```python
from build123d import *

# Parameters (mm, degrees)
SKETCH1_W               = 212.5
SKETCH1_H               = 339.725
BOSS_EXTRUDE1_DEPTH     = 6
SKETCH2_W               = 6.5
SKETCH2_H               = 20
BOSS_EXTRUDE2_DEPTH     = 24
CUT_EXTRUDE1_DEPTH      = 393.36344838
CUT_EXTRUDE1_DEPTH_BACK = 393.36344838
SKETCH3_R               = 4
FILLET2_R               = 5
SKETCH5_R               = 3.175
CUT_EXTRUDE2_DEPTH      = 402.314497153
CUT_EXTRUDE3_DEPTH      = 402.314497153


with BuildPart() as part:
    # Sketch1 → Boss-Extrude1 (new body)
    with BuildSketch(Plane.XY):
        with Locations((106.25, -169.8625)):
            Rectangle(SKETCH1_W, SKETCH1_H)
    extrude(amount=BOSS_EXTRUDE1_DEPTH)

    # Sketch2 → Boss-Extrude2 (add)
    with BuildSketch(Plane.XY.offset(6)):
        with Locations((21.75, -35.2425)):
            Rectangle(SKETCH2_W, SKETCH2_H)
        with Locations((50.75, -35.2425)):
            Rectangle(SKETCH2_W, SKETCH2_H)
        with Locations((190.75, -35.2425)):
            Rectangle(SKETCH2_W, SKETCH2_H)
        with Locations((161.75, -35.2425)):
            Rectangle(SKETCH2_W, SKETCH2_H)
        with Locations((133.75, -104.5325)):
            Rectangle(SKETCH2_W, SKETCH2_H)
        with Locations((165.25, -104.5325)):
            Rectangle(SKETCH2_W, SKETCH2_H)
        with Locations((165.25, -235.1925)):
            Rectangle(SKETCH2_W, SKETCH2_H)
        with Locations((21.75, -304.4825)):
            Rectangle(SKETCH2_W, SKETCH2_H)
        with Locations((50.75, -304.4825)):
            Rectangle(SKETCH2_W, SKETCH2_H)
        with Locations((190.75, -304.4825)):
            Rectangle(SKETCH2_W, SKETCH2_H)
        with Locations((161.75, -304.4825)):
            Rectangle(SKETCH2_W, SKETCH2_H)
        with Locations((133.75, -235.1925)):
            Rectangle(SKETCH2_W, SKETCH2_H)
    extrude(amount=BOSS_EXTRUDE2_DEPTH)

    # Sketch3 → Cut-Extrude1 (cut, two sides: drawn at the far end of the back side and taken through both)
    with BuildSketch(Plane.ZY.offset(-18.5).offset(-CUT_EXTRUDE1_DEPTH_BACK)):
        with Locations(Location((18, -35.2425, 0), (0, 0, 180))):
            Circle(SKETCH3_R)
        with Locations((18, -235.1925)):
            Circle(SKETCH3_R)
        with Locations(Location((18, -304.4825, 0), (0, 0, 270))):
            Circle(SKETCH3_R)
        with Locations(Location((18, -104.5325, 0), (0, 0, 180))):
            Circle(SKETCH3_R)
        with BuildLine():
            Line((18, -25.2425), (18, -12.982943413))
            Line((18, -12.982943413), (51.949532367, -12.982943413))
            Line((51.949532367, -12.982943413), (51.949532367, -57.481006387))
            Line((51.949532367, -57.481006387), (18, -57.481006387))
            Line((18, -57.481006387), (18, -45.2425))
            ThreePointArc((18, -45.2425), (28, -35.2425), (18, -25.2425))
        make_face()
        with BuildLine():
            Line((52.442304634, -132.399123951), (18, -132.399123951))
            Line((18, -132.399123951), (18, -114.5325))
            ThreePointArc((18, -114.5325), (28, -104.5325), (18, -94.5325))
            Line((18, -94.5325), (18, -71.59149594))
            Line((18, -71.59149594), (52.442304634, -71.59149594))
            Line((52.442304634, -71.59149594), (52.442304634, -132.399123951))
        make_face()
        with BuildLine():
            Line((52.599532243, -270.375386727), (18, -270.375386727))
            Line((18, -270.375386727), (18, -245.1925))
            ThreePointArc((18, -245.1925), (28, -235.1925), (18, -225.1925))
            Line((18, -225.1925), (18, -207.306351849))
            Line((18, -207.306351849), (52.599532243, -207.306351849))
            Line((52.599532243, -207.306351849), (52.599532243, -270.375386727))
        make_face()
        with BuildLine():
            Line((52.621034016, -326.721115515), (18, -326.721115515))
            Line((18, -326.721115515), (18, -314.4825))
            ThreePointArc((18, -314.4825), (28, -304.4825), (18, -294.4825))
            Line((18, -294.4825), (18, -282.222834285))
            Line((18, -282.222834285), (52.621034016, -282.222834285))
            Line((52.621034016, -282.222834285), (52.621034016, -326.721115515))
        make_face()
    extrude(amount=CUT_EXTRUDE1_DEPTH + CUT_EXTRUDE1_DEPTH_BACK, mode=Mode.SUBTRACT)

    # Fillet2
    fillet2_edges = [part.edges().sort_by_distance(p)[0] for p in [
        (190.75, -45.2425, 6),
        (194, -35.2425, 6),
        (190.75, -25.2425, 6),
        (50.75, -45.2425, 6),
        (54, -35.2425, 6),
        (50.75, -25.2425, 6),
        (21.75, -25.2425, 6),
        (18.5, -35.2425, 6),
        (21.75, -45.2425, 6),
        (161.75, -25.2425, 6),
        (158.5, -35.2425, 6),
        (161.75, -45.2425, 6),
        (161.75, -294.4825, 6),
        (161.75, -314.4825, 6),
        (158.5, -304.4825, 6),
        (190.75, -314.4825, 6),
        (194, -304.4825, 6),
        (190.75, -294.4825, 6),
        (165.25, -245.1925, 6),
        (168.5, -235.1925, 6),
        (165.25, -225.1925, 6),
        (133.75, -225.1925, 6),
        (130.5, -235.1925, 6),
        (133.75, -245.1925, 6),
        (50.75, -314.4825, 6),
        (54, -304.4825, 6),
        (50.75, -294.4825, 6),
        (21.75, -294.4825, 6),
        (21.75, -314.4825, 6),
        (18.5, -304.4825, 6),
        (165.25, -114.5325, 6),
        (165.25, -94.5325, 6),
        (168.5, -104.5325, 6),
        (133.75, -94.5325, 6),
        (130.5, -104.5325, 6),
        (133.75, -114.5325, 6),
    ]]
    fillet(fillet2_edges, radius=FILLET2_R)

    # Sketch5 → Cut-Extrude2 (cut, through all)
    with BuildSketch(Plane.XY.offset(6)):
        with Locations((12.7, -12.7)):
            Circle(SKETCH5_R)
        with Locations((199.8, -12.7)):
            Circle(SKETCH5_R)
        with Locations((66.25, -35.2425)):
            Circle(SKETCH5_R)
        with Locations((146.25, -35.2425)):
            Circle(SKETCH5_R)
        with Locations((176.25, -57.8625)):
            Circle(SKETCH5_R)
        with Locations((36.25, -57.8625)):
            Circle(SKETCH5_R)
        with Locations((191.25, -104.5325)):
            Circle(SKETCH5_R)
        with Locations((36.25, -169.8625)):
            Circle(SKETCH5_R)
        with Locations((191.25, -169.8625)):
            Circle(SKETCH5_R)
        with Locations((36.25, -281.8625)):
            Circle(SKETCH5_R)
        with Locations((66.25, -304.4825)):
            Circle(SKETCH5_R)
        with Locations((12.7, -327.025)):
            Circle(SKETCH5_R)
        with Locations((199.8, -327.025)):
            Circle(SKETCH5_R)
        with Locations((146.25, -304.4825)):
            Circle(SKETCH5_R)
        with Locations(Location((191.25, -235.1925, 0), (0, 0, 180))):
            Circle(SKETCH5_R)
    extrude(amount=-CUT_EXTRUDE2_DEPTH, mode=Mode.SUBTRACT)

    # Sketch9 → Cut-Extrude3 (cut, through all)
    with BuildSketch(Plane.XY.offset(6)):
        with BuildLine():
            Line((70, -271.3625), (110, -271.3625))
            ThreePointArc((110, -271.3625), (114.242640687, -269.605140687), (116, -265.3625))
            Line((116, -265.3625), (116, -74.3625))
            ThreePointArc((116, -74.3625), (114.242640687, -70.119859313), (110, -68.3625))
            Line((110, -68.3625), (70, -68.3625))
            ThreePointArc((70, -68.3625), (65.757359313, -70.119859313), (64, -74.3625))
            Line((64, -74.3625), (64, -265.3625))
            ThreePointArc((64, -265.3625), (65.757359313, -269.605140687), (70, -271.3625))
        make_face()
    extrude(amount=-CUT_EXTRUDE3_DEPTH, mode=Mode.SUBTRACT)


solid = part.part
```
Part model, mm, in its own coordinate system. A direction names the side the tool comes from. Coordinates: 2 decimals unless noted, no trailing zeros. Order: outer loops, then holes, each group sorted by start corner. A loop starts at its lowest first (then second) coordinate and runs counter-clockwise, first axis right, second up. Notation, with made-up numbers: (-34.75, 76.25) - (-11.75, 76.25) arc R11 ccw to (-11.75, 96.25) - close; hole circle Ø5 at (-12.75, 33.25). An arc over 180 degrees is marked (long way). Return JSON: item names as keys, results as strings. Group by question number.
Item 1: Pin check, flat tips, straight feed: pin 1 (7 mm diameter, centred on x = 162.5, z = 14.5, fed in from -Y); pin 2 (13.5 mm diameter, centred on y = -235.5, z = 21, fed in from -X); pin 3 (9 mm diameter, centred on y = -35.24, z = 18, fed in from +X); pin 4 (1.5 mm diameter, centred on x = 140, y = -176, fed in from -Z). Stop position of each tip, or through.
Item 2: Cut at B-B (x = 106.5). List the corners of the cut face in (y, z) (1 decimal), plus the area to 3 significant figures.
Item 3: Drill centre lines: probe 1 along Y at (x, z) = (36.25, 2.5) (1 decimal); probe 2 along Y at (x, z) = (20.25, 18); probe 3 along Y at (x, z) = (12.7, 1.8) (3 decimals). Where is each one in solid material? Low to high. Write a range as from..to.
Item 4: Pull direction X, two halves, no side cores. Call faces 6 (the face through (190.796, -304.702, 27.998)), 7 (the face through (162, -232, 14)): pulls with the +X half, pulls with the -X half, needs draft (parallel to the pull), parting line crosses it, or undercut.
Item 5: Cut at A-A (y = -130). List the corners of the cut face in (x, z), plus the area to 3 significant figures.
Item 6: Which spindle directions (+Z, -Z, +X, -X, +Y, -Y) get a long thin tool onto all of the face, cutting with end or side? Do faces 1 (the face through (161.796, -32.809, 21.174)), 2 (the face through (54, -31, 19)), 3 (the face through (162, -294.482, 14)), 4 (the face through (134, -94.532, 14)), 5 (the face through (162, -101, 14)). Say none if no direction does.
Check values:
{
 "1": {"pin 1": "stops at y = -314.48", "pin 2": "stops at x = 130.5", "pin 3": "stops at x = 194", "pin 4": "stops at z = 0"},
 "2": {"outline": "(-339.7, 0) - (-271.4, 0) - (-271.4, 6) - (-339.7, 6) - close; (-68.4, 0) - (0, 0) - (0, 6) - (-68.4, 6) - close", "area": "820 mm2"},
 "3": {"probe 1": "y = -339.7..-285, -278.7..-173, -166.7..-61, -54.7..0", "probe 2": "y = -314.48..-308.48, -300.48..-294.48, -45.24..-39.24, -31.24..-25.24", "probe 3": "y = -339.725..-330.2, -323.85..-15.875, -9.525..0"},
 "4": {"face 6": "needs draft", "face 7": "undercut"},
 "5": {"outline": "(0, 0) - (64, 0) - (64, 6) - (0, 6) - close; (116, 0) - (212.5, 0) - (212.5, 6) - (116, 6) - close", "area": "963 mm2"},
 "6": {"face 1": "+X, -X", "face 2": "+Z, +Y, -Y", "face 3": "+Z, +X, -X", "face 4": "+Z, +X, -X, +Y", "face 5": "+Z"}
}
